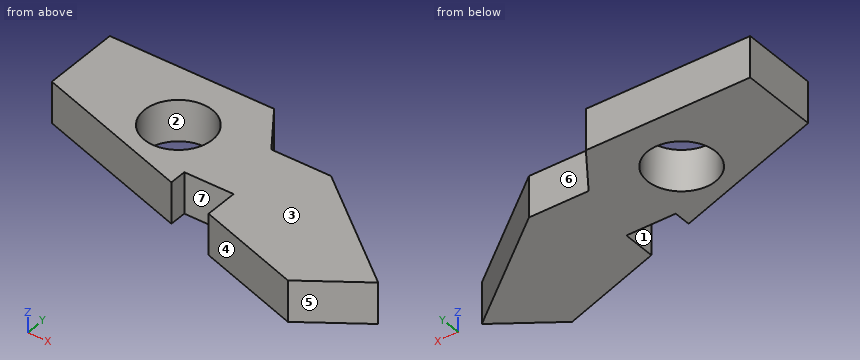
```python
from build123d import *

# Parameters (mm, degrees)
F0_R     = 20.650095
F1_DEPTH = 25
F2_W     = 30
F2_H     = 32.013418
F3_DEPTH = 25


with BuildPart() as f1:
    # F0 (on Top) → F1 (new body)
    with BuildSketch(Plane.XY):
        Polygon((29.359795, 67.968812), (-70.640205, 67.968812), (-70.640205, 20.943799), (119.507518, -41.054939), (155.728, -16.081285), (84.712092, 40.356558), (48.398163, 40.356558), align=None)
        with Locations((0, 29.416777)):
            Circle(F0_R, mode=Mode.SUBTRACT)
    extrude(amount=F1_DEPTH)

    # F2 (on Top) → F3 (cut)
    with BuildSketch(Plane.XY):
        with Locations((40.671138, -16.006709)):
            Rectangle(F2_W, F2_H)
    extrude(amount=F3_DEPTH, mode=Mode.SUBTRACT)


solid = f1.part
```
Geometry: final body of the model. Coordinates: model frame, mm. Face numbers are marked on the shaded views. A direction names the side the tool comes from. Coordinates: 2 decimals unless noted, no trailing zeros. Order: outer loops, then holes, each group sorted by start corner. A loop starts at its lowest first (then second) coordinate and runs counter-clockwise, first axis right, second up. Notation, with made-up numbers: (88, 73.25) - (95, 73.25) arc R23 cw to (95, 97.25) - close; hole circle Ø3 at (66.25, 75.5). An arc over 180 degrees is marked (long way). Return JSON: item names as keys, results as strings. Group by question number.
1. Cut plane D-D (x = 66). Output: boundary loops of the cut face in (y, z).
2. Cut plane C-C (z = 14). Output: boundary loops of the cut face in (x, y), plus the area to 3 significant figures.
3. Cut plane A-A (x = -15.5). Output: boundary loops of the cut face in (y, z), plus the area to 3 significant figures.
4. Material intervals for line 1 along Y through (x, z) = (0, 5.5); line 2 along X through (y, z) = (46.5, 19.75); line 3 along X through (y, z) = (52, 4.75), sorted ascending. Write a range as [from, to].
5. Cut plane B-B (y = 11). Output: boundary loops of the cut face in (x, z), plus the area to 3 significant figures.
6. Pin query (flat end, axial travel): pin 1 (7.5 mm diameter, centred on x = 45, z = 18.5, fed in from -Y); pin 2 (2 mm diameter, centred on x = -1, z = 17.5, fed in from -Y); pin 3 (5 mm diameter, centred on y = -3, z = 9.5, fed in from +X). Return the tip coordinate at first contact, or that it passes through.
7. Pull-direction query (X, two-part tool) for the marked faces 1, 2, 3 and 4; classes: pulls with the +X half, pulls with the -X half, needs draft (parallel to the pull), parting line crosses it, or undercut.
8. Set-up query: the marked faces 5, 6 and 7. Return all of +Z, -Z, +X, -X, +Y, -Y with unobstructed straight access to the full face (end or side cutting, diameter ignored); none if empty.
Resolved:
{
 "1": {"outline": "(-23.61, 0) - (40.36, 0) - (40.36, 25) - (-23.61, 25) - close"},
 "2": {"outline": "(-70.64, 20.94) - (25.67, -10.46) - (25.67, 0) - (55.67, 0) - (55.67, -20.24) - (119.51, -41.05) - (155.73, -16.08) - (84.71, 40.36) - (48.4, 40.36) - (29.36, 67.97) - (-70.64, 67.97) - close; hole circle Ø41.3 at (0, 29.42)", "area": "11,300 mm²"},
 "3": {"outline": "(2.97, 0) - (15.77, 0) - (15.77, 25) - (2.97, 25) - close; (43.06, 0) - (67.97, 0) - (67.97, 25) - (43.06, 25) - close", "area": "943 mm²"},
 "4": {"line 1": "y = [-2.09, 8.77], [50.07, 67.97]", "line 2": "x = [-70.64, -11.6], [11.6, 44.16]", "line 3": "x = [-70.64, 40.37]"},
 "5": {"outline": "(-40.14, 0) - (-9.34, 0) - (-9.34, 25) - (-40.14, 25) - close; (9.34, 0) - (121.65, 0) - (121.65, 25) - (9.34, 25) - close", "area": "3,580 mm²"},
 "6": {"pin 1": "stops at y = 0", "pin 2": "stops at y = -2.09", "pin 3": "stops at x = 142.41"},
 "7": {"face 1": "undercut", "face 2": "undercut", "face 3": "needs draft", "face 4": "pulls with the -X half"},
 "8": {"face 5": "+Z, -Z, +X, -Y", "face 6": "+Z, -Z, +X, +Y", "face 7": "+Z, -Z, -Y"}
}
